The figure shows three views and two pictorial views of one solid part (mm, origin at its lowest corner). Answer the questions. A direction names the side the tool comes from. Round coordinates to 2 decimals unless told otherwise and drop trailing zeros. Loops run counter-clockwise (first coordinate to the right, second up) from the corner with the lowest first, then second, coordinate; pieces in that order, holes last. Notation, with made-up numbers: (67.25, 80) -> (91.25, 80) arc R18 cw to (91.25, 94) -> close; hole circle Ø4 at (79, 2). An arc over 180 degrees is marked (long way). Use a Markdown table: item, result. Add a question column.
Q1. Consider line 1 (X direction, y = 0.5, z = 25); line 2 (Z direction, x = 10, y = 1). Determine where each line is inside the solid, lowest interval first.
Q2. Section A-A on z = 25 is taken. Give the vertices of the cut face in (x, y).
Q3. Given pin 1 Ø10 at (x, y) = (16.5, 18) entering from +Z; pin 2 Ø6 at (x, z) = (8, 31) entering from +Y, each flat-ended and moving along its own axis, determine where each tip first touches the part or whether it passes through.
Q4. Which of the six approach directions +Z, -Z, +X, -X, +Y, -Y give full straight-line access (tool end or side, diameter ignored) to the marked faces 1 and 2?
Q5. Section D-D on y = 11 is taken. Give the vertices of the cut face in (x, z).
Q6. Section B-B on x = 10 is taken. Give the vertices of the cut face in (y, z).
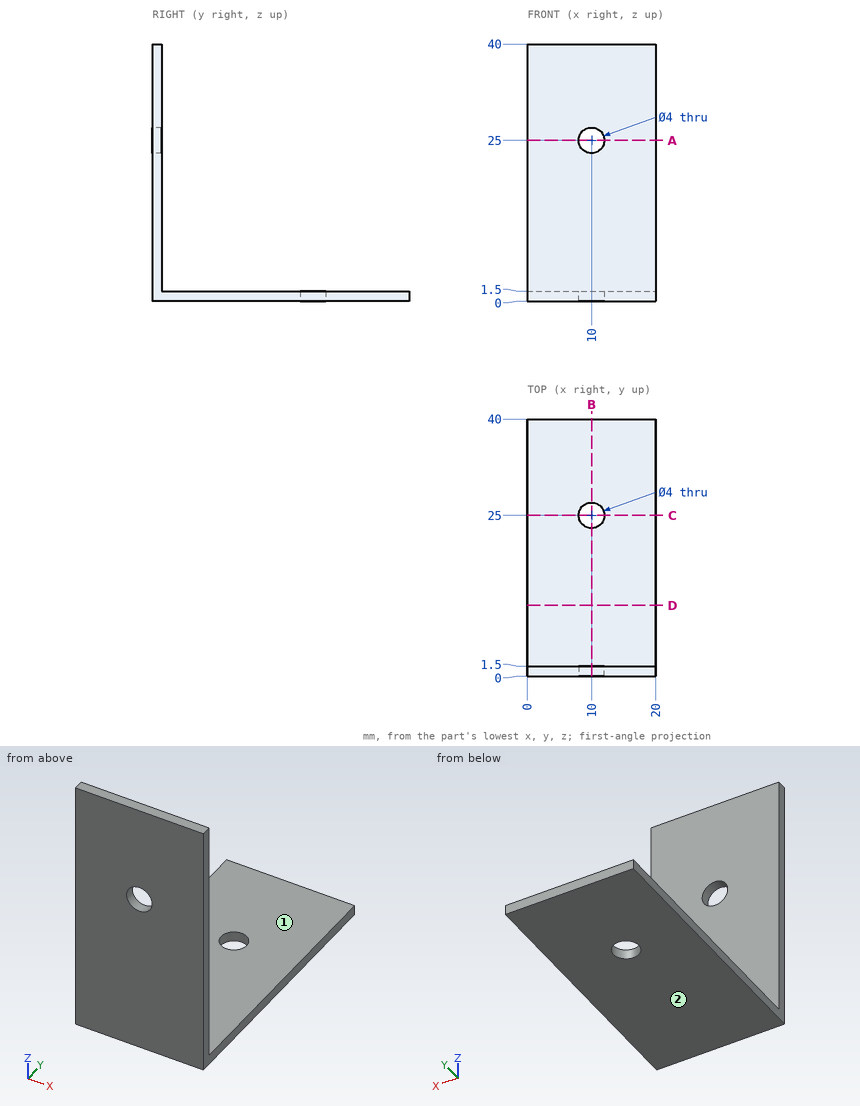
Checked values:
| question | item | result |
|---|---|---|
| 1 | line 1 | x = 0 to 8, 12 to 20 |
| 1 | line 2 | z = 0 to 23, 27 to 40 |
| 2 | outline | (0, 0) -> (8, 0) -> (8, 1.5) -> (0, 1.5) -> close; (12, 0) -> (20, 0) -> (20, 1.5) -> (12, 1.5) -> close |
| 3 | pin 1 | stops at z = 1.5 |
| 3 | pin 2 | stops at y = 1.5 |
| 4 | face 1 | +Z, +X, -X, +Y |
| 4 | face 2 | -Z, +X, -X, +Y, -Y |
| 5 | outline | (0, 0) -> (20, 0) -> (20, 1.5) -> (0, 1.5) -> close |
| 6 | outline | (0, 0) -> (23, 0) -> (23, 1.5) -> (1.5, 1.5) -> (1.5, 23) -> (0, 23) -> close; (0, 27) -> (1.5, 27) -> (1.5, 40) -> (0, 40) -> close; (27, 0) -> (40, 0) -> (40, 1.5) -> (27, 1.5) -> close |
